Study the drawing (mm; zero at the part's minimum x, y, z) and answer. A direction names the side the tool comes from. Round coordinates to 2 decimals unless told otherwise and drop trailing zeros. Order: outer loops, then holes, each group sorted by start corner. A loop starts at its lowest first (then second) coordinate and runs counter-clockwise, first axis right, second up. Notation, with made-up numbers: (15.25, 81) - (24.25, 81) arc R15 ccw to (24.25, 99) - close; hole circle Ø4 at (-27.5, -20.5). An arc over 180 degrees is marked (long way). Put each result on its own line as item: value. Start each with the question number.
Q1. Which of the six approach directions +Z, -Z, +X, -X, +Y, -Y give full straight-line access (tool end or side, diameter ignored) to the marked faces 1, 2 and 3?
Q2. Section B-B on z = 41.5 is taken. Give the vertices of the cut face in (x, y), then the cut area to 3 significant figures.
Q3. Find the intervals of material crossed by line 1 along Y through (x, z) = (18.1, 41.5); line 2 along Z through (x, y) = (15.75, 21.25); line 3 along X through (y, z) = (25, 7), in increasing order. Write a range as from..to.
Q4. Section C-C on y = 14.25 is taken. Give the vertices of the cut face in (x, z).
Q5. Section A-A on y = 4 is taken. Give the vertices of the cut face in (x, z), then the cut area to 3 significant figures.
Q6. Section D-D on x = 15.25 is taken. Give the vertices of the cut face in (y, z).
Q7. Each of these flat-tipped pins is pushed along its axis until it touches: pin 1 Ø5.5 at (y, z) = (4, 58.5) entering from -X; pin 2 Ø8 at (y, z) = (15, 75.5) entering from -X; pin 3 Ø5 at (y, z) = (18.5, 80.5) entering from +X. Where does it stop, or does it pass through?
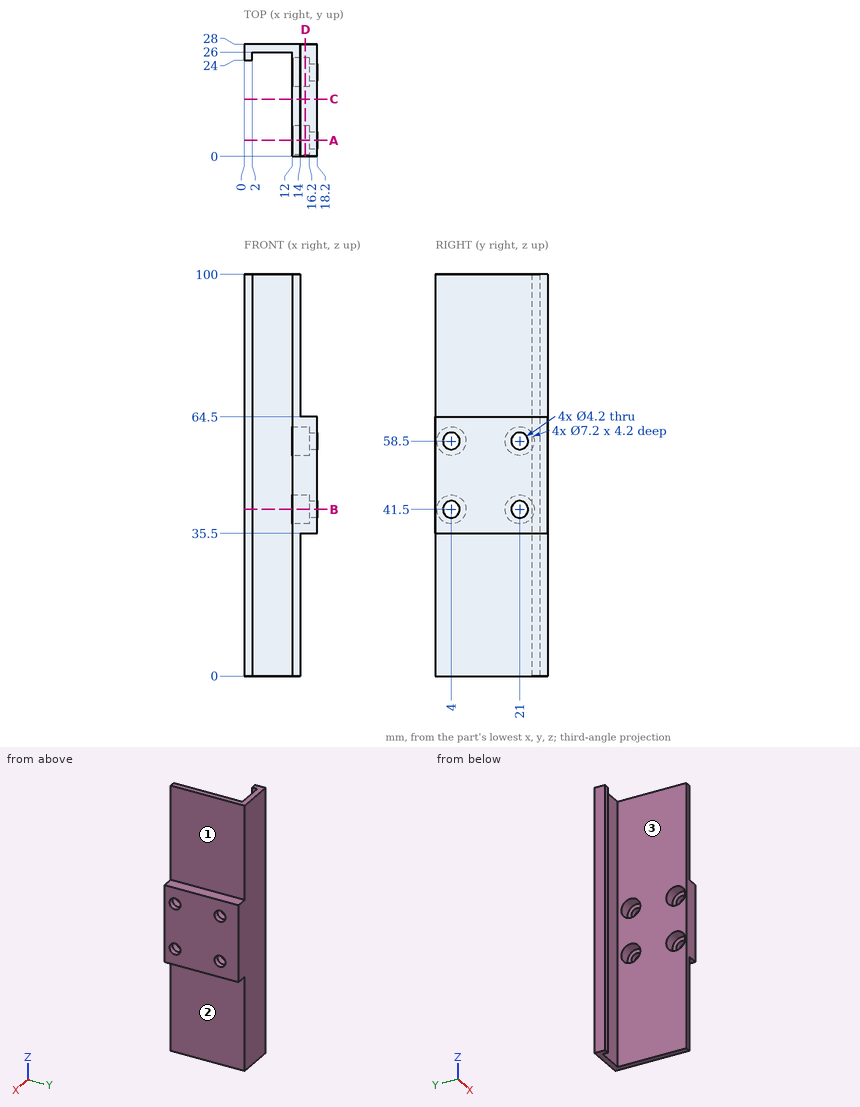
Findings:
1. face 1: +Z, +X, +Y, -Y
1. face 2: -Z, +X, +Y, -Y
1. face 3: +Z, -Z, -Y
2. outline: (0, 24) - (2, 24) - (2, 26) - (12, 26) - (12, 24.6) - (16.2, 24.6) - (16.2, 23.1) - (18.2, 23.1) - (18.2, 28) - (0, 28) - close; (12, 0) - (18.2, 0) - (18.2, 1.9) - (16.2, 1.9) - (16.2, 0.4) - (12, 0.4) - close; (12, 7.6) - (16.2, 7.6) - (16.2, 6.1) - (18.2, 6.1) - (18.2, 18.9) - (16.2, 18.9) - (16.2, 17.4) - (12, 17.4) - close
2. area: 124 mm2
3. line 1: 0..1.9, 6.1..18.9, 23.1..28
3. line 2: 35.5..37.91, 45.09..54.91, 62.09..64.5
3. line 3: 0..2, 12..14
4. outline: (12, 0) - (14, 0) - (14, 35.5) - (18.2, 35.5) - (18.2, 64.5) - (14, 64.5) - (14, 100) - (12, 100) - close
5. outline: (12, 0) - (14, 0) - (14, 35.5) - (18.2, 35.5) - (18.2, 39.4) - (16.2, 39.4) - (16.2, 37.9) - (12, 37.9) - close; (12, 45.1) - (16.2, 45.1) - (16.2, 43.6) - (18.2, 43.6) - (18.2, 56.4) - (16.2, 56.4) - (16.2, 54.9) - (12, 54.9) - close; (12, 62.1) - (16.2, 62.1) - (16.2, 60.6) - (18.2, 60.6) - (18.2, 64.5) - (14, 64.5) - (14, 100) - (12, 100) - close
5. area: 245 mm2
6. outline: (0, 35.5) - (28, 35.5) - (28, 64.5) - (0, 64.5) - close; hole circle Ø7.2 at (4, 41.5); hole circle Ø7.2 at (4, 58.5); hole circle Ø7.2 at (21, 41.5); hole circle Ø7.2 at (21, 58.5)
7. pin 1: x = 16.2
7. pin 2: x = 12
7. pin 3: x = 14
